Can you work these out from the model? Positions are in its coordinate system, mm. A direction names the side the tool comes from. Coordinates: 2 decimals unless noted, no trailing zeros. Write each loop counter-clockwise with the first axis right and the second up, starting at its lowest first coordinate (ties: lowest second). Pieces come first, ordered by that corner, then holes. Notation, with made-up numbers: (6, 65) -> (62, 65) arc R24 ccw to (62, 87) -> close; hole circle Ø11 at (59, 12.5). An arc over 180 degrees is marked (long way). Use one line per item in the form item = value.
```python
from build123d import *

# Parameters (mm, degrees)
SKETCH1_W                 = 76.2
SKETCH1_H                 = 88.9
BOSS_EXTRUDE1_DEPTH       = 4.7625
F_8_CLEARANCE_HOLE1_D     = 4.4958
FILLET1_R                 = 2.54
F_8_CLEARANCE_SLOT1_DEPTH = 4.7625
SKETCH6_R                 = 4.064
CUT_EXTRUDE1_DEPTH        = 64.678343306
F_8_CLEARANCE_HOLE2_D     = 4.4958
SKETCH9_R                 = 2.2479
BOSS_EXTRUDE2_DEPTH       = 4.7625


# Read off the part's stored shape, not the designer's step: #8 Clearance Slot1
with BuildPart() as part:
    # Sketch1 → Boss-Extrude1 (new body)
    with BuildSketch(Plane.XY):
        with Locations((0, 6.35)):
            Rectangle(SKETCH1_W, SKETCH1_H)
    extrude(amount=BOSS_EXTRUDE1_DEPTH)

    # #8 Clearance Hole1 (through all)
    with Locations(Plane.XY.offset(4.7625)):
        with Locations((23.57, 23.57), (-23.57, 23.755), (23.57, -23.57), (-23.57, -23.57)):
            Hole(F_8_CLEARANCE_HOLE1_D / 2)

    # Fillet1
    fillet1_edges = [part.edges().sort_by_distance(p)[0] for p in [
        (-38.1, 50.8, 2.38125),
        (38.1, 50.8, 2.38125),
        (38.1, -38.1, 2.38125),
        (-38.1, -38.1, 2.38125),
    ]]
    fillet(fillet1_edges, radius=FILLET1_R)

    # #8 Clearance Slot1 outline → #8 Clearance Slot1 (cut)
    with BuildSketch(Plane.XY):
        with BuildLine():
            ThreePointArc((-27.55265, 39.61765), (-25.4, 37.465), (-23.24735, 39.61765))
            Line((-23.24735, 39.61765), (-23.24735, 44.83735))
            ThreePointArc((-23.24735, 44.83735), (-25.4, 46.99), (-27.55265, 44.83735))
            Line((-27.55265, 44.83735), (-27.55265, 39.61765))
        make_face()
        with BuildLine():
            ThreePointArc((23.24735, 39.61765), (25.4, 37.465), (27.55265, 39.61765))
            Line((27.55265, 39.61765), (27.55265, 44.83735))
            ThreePointArc((27.55265, 44.83735), (25.4, 46.99), (23.24735, 44.83735))
            Line((23.24735, 44.83735), (23.24735, 39.61765))
        make_face()
    extrude(amount=F_8_CLEARANCE_SLOT1_DEPTH, mode=Mode.SUBTRACT)

    # Sketch6 → Cut-Extrude1 (cut, through all)
    with BuildSketch(Plane(origin=(0, 0, 0), x_dir=(-1, 0, 0), z_dir=(0, 0, -1))):
        with Locations((-25.4, 39.61765)):
            Circle(SKETCH6_R)
        with Locations((25.4, 39.61765)):
            Circle(SKETCH6_R)
    extrude(amount=-CUT_EXTRUDE1_DEPTH, mode=Mode.SUBTRACT)

    # #8 Clearance Hole2 (through all)
    with Locations(Plane(origin=(0, 0, 0), x_dir=(-1, 0, 0), z_dir=(0, 0, -1))):
        with Locations((31.75, 31.75), (31.75, -31.75), (-31.75, -31.75), (-31.75, 31.75)):
            Hole(F_8_CLEARANCE_HOLE2_D / 2)

    # Sketch9 → Boss-Extrude2 (add, through all)
    # profile 1 of 2: a face of its own
    with BuildSketch(Plane.XY.offset(4.7625)):
        with BuildLine():
            Line((-38.1, -43.18), (-38.1, -35.56))
            Line((-38.1, -35.56), (-25.4, -35.56))
            Line((-25.4, -35.56), (-25.4, -43.18))
            ThreePointArc((-25.4, -43.18), (-31.75, -49.53), (-38.1, -43.18))
        make_face()
        with Locations((-31.75, -43.18)):
            Circle(SKETCH9_R, mode=Mode.SUBTRACT)
    # profile 2 of 2: a face of its own
    with BuildSketch(Plane.XY.offset(4.7625)):
        with BuildLine():
            Line((25.4, -35.56), (25.4, -43.18))
            ThreePointArc((25.4, -43.18), (31.75, -49.53), (38.1, -43.18))
            Line((38.1, -43.18), (38.1, -35.56))
            Line((38.1, -35.56), (25.4, -35.56))
        make_face()
        with Locations((31.75, -43.18)):
            Circle(SKETCH9_R, mode=Mode.SUBTRACT)
    extrude(amount=-BOSS_EXTRUDE2_DEPTH)


solid = part.part
```
Q1. If I drill on line 1 (X direction, y = -32, z = 0.5); line 2 (Y direction, x = 31.75, z = 3.35); line 3 (X direction, y = 46.5, z = 0.55), over which ranges is the centre line in solid material (lowest first)? Write a range as from..to.
Return value:
line_1 = -38.1..-33.98, -29.52..29.52, 33.98..38.1
line_2 = -49.53..-45.43, -40.93..-34, -29.5..29.5, 34..50.8
line_3 = -38.1..-26.77, -24.03..24.03, 26.77..38.1
Q2. Suppose I cut it at A-A (y = -31.75). Write out the boundary of the cut face in (x, z).
Return value:
outline = (-38.1, 0) -> (-34, 0) -> (-34, 4.76) -> (-38.1, 4.76) -> close; (-29.5, 0) -> (29.5, 0) -> (29.5, 4.76) -> (-29.5, 4.76) -> close; (34, 0) -> (38.1, 0) -> (38.1, 4.76) -> (34, 4.76) -> close
Q3. Suppose I cut it at C-C (z = 3.9). Give the number of separate pieces and of enclosed holes in the cut face, then the cut area to 3 significant figures.
Return value:
separate_pieces = 1
enclosed_holes = 12
area = 6,740 mm2
Q4. Suppose I cut it at D-D (x = -5). Write out the boundary of the cut face in (y, z), then the cut area to 3 significant figures.
Return value:
outline = (-38.1, 0) -> (50.8, 0) -> (50.8, 4.76) -> (-38.1, 4.76) -> close
area = 423 mm2
Q5. For faces 1 (the cylindrical face through (25.45, 46.99, 2.35)), 2 (the flat face through (0, 50.8, 2)), 3 (the flat face through (0, -38.1, 2)), which set-ups out of +Z, -Z, +X, -X, +Y, -Y let a thin tool reach every point of the face, with its end or its side?
Return value:
face_1 = +Z, -Z
face_2 = +Z, -Z, +X, -X, +Y
face_3 = +Z, -Z, -Y
Q6. Thinking about a two-plate mould opening in X: for faces 4 (the flat face through (1, 1, 0)), 5 (the flat face through (-25.4, -41, 2)), 6 (the flat face through (-38.1, 2, 2)), which applies, released by +X, released by -X, zero draft, split by the parting line, or undercut?
Return value:
face_4 = zero draft
face_5 = undercut
face_6 = released by -X
Q7. Suppose I cut it at B-B (x = -31.75). Write out the boundary of the cut face in (y, z), then the cut area to 3 significant figures.
Return value:
outline = (-49.53, 0) -> (-45.43, 0) -> (-45.43, 4.76) -> (-49.53, 4.76) -> close; (-40.93, 0) -> (-34, 0) -> (-34, 4.76) -> (-40.93, 4.76) -> close; (-29.5, 0) -> (29.5, 0) -> (29.5, 4.76) -> (-29.5, 4.76) -> close; (34, 0) -> (50.8, 0) -> (50.8, 4.76) -> (34, 4.76) -> close
area = 414 mm2
